```python
from build123d import *

# Parameters (mm, degrees)
SKETCH1_W                   = 555.625
SKETCH1_H                   = 298.45
BOSS_EXTRUDE1_DEPTH         = 3.175
SKETCH2_W                   = 9.525
SKETCH2_H                   = 203.2
CUT_EXTRUDE1_DEPTH          = 4.175
FILLET1_R                   = 3.175
F_1_4_0_25_DIAMETER_HOLE1_D = 6.35
FILLET2_R                   = 3.175


with BuildPart() as part:
    # Sketch1 → Boss-Extrude1 (new body)
    with BuildSketch(Plane(origin=(0, 0, 0), x_dir=(1, 0, 0), z_dir=(0, 1, 0))):
        Rectangle(SKETCH1_W, SKETCH1_H)
    extrude(amount=BOSS_EXTRUDE1_DEPTH)

    # Sketch2 → Cut-Extrude1 (cut, through all)
    with BuildSketch(Plane(origin=(0, 3.175, 0), x_dir=(1, 0, 0), z_dir=(0, 1, 0))):
        with Locations((273.05, 0)):
            Rectangle(SKETCH2_W, SKETCH2_H)
    extrude(amount=-CUT_EXTRUDE1_DEPTH, mode=Mode.SUBTRACT)

    # Fillet1
    fillet1_edges = [part.edges().sort_by_distance(p)[0] for p in [
        (268.2875, 1.5875, 101.6),
        (268.2875, 1.5875, -101.6),
    ]]
    fillet(fillet1_edges, radius=FILLET1_R)

    # 1/4 (0.25) Diameter Hole1 (through all)
    with Locations(Plane(origin=(0, 0, 0), x_dir=(-1, 0, 0), z_dir=(0, -1, 0))):
        with Locations((-167.5765, -142.875), (214.3125, -142.875)):
            f_1_4_0_25_diameter_hole1 = Hole(F_1_4_0_25_DIAMETER_HOLE1_D / 2)

    # Mirror1: 1/4 (0.25) Diameter Hole1 across plane
    add(f_1_4_0_25_diameter_hole1.mirror(Plane.XY), mode=Mode.SUBTRACT)

    # Fillet2
    fillet2_edges = [part.edges().sort_by_distance(p)[0] for p in [
        (277.8125, 1.5875, -101.6),
        (277.8125, 1.5875, 101.6),
        (277.8125, 1.5875, 149.225),
        (-277.8125, 1.5875, 149.225),
        (-277.8125, 1.5875, -149.225),
        (277.8125, 1.5875, -149.225),
    ]]
    fillet(fillet2_edges, radius=FILLET2_R)


solid = part.part
```
CAD build for the part. Positions are in the model's coordinates, mm. Coordinates: 2 decimals unless noted, no trailing zeros. Write each loop counter-clockwise with the first axis right and the second up, starting at its lowest first coordinate (ties: lowest second). Pieces come first, ordered by that corner, then holes. Notation, with made-up numbers: (40.5, 35.25) -> (71.5, 35.25) arc R20 ccw to (71.5, 51.25) -> close; hole circle Ø10 at (36.5, -36.5). An arc over 180 degrees is marked (long way). Use CSV: the item, a comma, the result in double quotes. Start each with the question number.
Item 1: Drop a flat-ended pin along its axis: P1, Ø1.6, axis at y = 1.5, z = -20, coming from the +X side. Give the stop position or say it passes through.
Item 2: Band-saw the part on A-A, the plane z = 65. Write the cut outline in (x, y) (1 decimal), plus the area to 3 significant figures.
Item 3: Wall check: probe 1 along X at (y, z) = (1.9, -3); probe 2 along Z at (x, y) = (-211.5, 2.8) (3 decimals); probe 3 along X at (y, z) = (1.7, -104). Give the ranges that are in metal, low to high.
Response values:
1,P1,"stops at x = 268.29"
2,outline,"(-277.8, 0) -> (268.3, 0) -> (268.3, 3.2) -> (-277.8, 3.2) -> close"
2,area,"1,730 mm2"
3,probe 1,"x = -277.81 to 268.29"
3,probe 2,"z = -149.225 to -144.348, -141.402 to 141.402, 144.348 to 149.225"
3,probe 3,"x = -277.81 to 277.72"
